```python
from build123d import *

# Parameters (mm, degrees)
SKETCH1_R                  = 20.6375
SKETCH1_R_2                = 17.4625
BOSS_EXTRUDE1_DEPTH        = 152.4
BOSS_EXTRUDE2_START        = -6.35
SKETCH2_R                  = 30.1625
SKETCH2_R_2                = 17.4625
BOSS_EXTRUDE2_DEPTH        = 6.35
F_10_32_TAPPED_HOLE1_D     = 4.0386
F_10_32_TAPPED_HOLE1_DEPTH = 6.35


with BuildPart() as part:
    # Sketch1 → Boss-Extrude1 (new body)
    with BuildSketch(Plane(origin=(0, 0, 0), x_dir=(1, 0, 0), z_dir=(0, 1, 0))):
        with Locations(Location((0, 0, 0), (0, 0, 90))):
            Circle(SKETCH1_R)
        with Locations(Location((0, 0, 0), (0, 0, 90))):
            Circle(SKETCH1_R_2, mode=Mode.SUBTRACT)
    extrude(amount=BOSS_EXTRUDE1_DEPTH)

    # Sketch2 → Boss-Extrude2 (add)
    with BuildSketch(Plane(origin=(0, 152.4, 0), x_dir=(1, 0, 0), z_dir=(0, 1, 0)).offset(BOSS_EXTRUDE2_START)):
        with Locations(Location((0, 0, 0), (0, 0, 270))):
            Circle(SKETCH2_R)
        with Locations(Location((0, 0, 0), (0, 0, 90))):
            Circle(SKETCH2_R_2, mode=Mode.SUBTRACT)
    extrude(amount=BOSS_EXTRUDE2_DEPTH)

    # #10-32 Tapped Hole1
    with Locations(Plane(origin=(0, 152.4, 0), x_dir=(1, 0, 0), z_dir=(0, 1, 0))):
        with Locations((-23.8125, 0), (0, 23.8125), (23.8125, 0), (0, -23.8125), (0, 0)):
            Hole(F_10_32_TAPPED_HOLE1_D / 2, depth=F_10_32_TAPPED_HOLE1_DEPTH)


solid = part.part
```
Here's how the part is built. I have some questions about the finished solid (model axes, mm). A direction names the side the tool comes from. Coordinates: 2 decimals unless noted, no trailing zeros. Write each loop counter-clockwise with the first axis right and the second up, starting at its lowest first coordinate (ties: lowest second). Pieces come first, ordered by that corner, then holes. Notation, with made-up numbers: (18, -26) -> (51, -26) arc R12 cw to (51, -10) -> close; hole circle Ø7 at (70, -31). An arc over 180 degrees is marked (long way). Use a Markdown table: item, result. Add a question column.
(1) If we section it at A-A, the plane z = 0: Write out the boundary of the cut face in (x, y), and give its area (3 significant figures).
(2) If we section it at B-B, the plane x = 11: Write out the boundary of the cut face in (y, z).
(3) Please list where these lines run through material, in increasing order: line 1 (Z direction, x = 0.5, y = 35); line 2 (Y direction, x = 24.5, z = -13); line 3 (Z direction, x = 5.5, y = 23).
(4) For faces 1 (the cylindrical face through (17, 75, 4)), 2 (the cylindrical face through (-20.46, 72, 2.69)), which set-ups out of +Z, -Z, +X, -X, +Y, -Y let a thin tool reach every point of the face, with its end or its side?
(5) If we section it at D-D, the plane x = -8: Write out the boundary of the cut face in (y, z), and give its area (3 significant figures).
(6) If we section it at C-C, the plane y = 82: Write out the boundary of the cut face in (x, z) (1 decimal), and give its area (3 significant figures).
(7) I'm going to push flat-ended pins straight in: P1, Ø10, axis at x = -20, y = 29, coming from the -Z side; P2, Ø5.5, axis at x = 0, z = 23.81, coming from the -Y side; P3, Ø3, axis at x = 10, y = 52, coming from the -Z side; P4, Ø5.5, axis at x = -23.81, z = 0, coming from the +Y side. Where does each tip first touch, or does it pass through?
(8) We'd pull the mould along X, two halves only. Please class faces 3 (the flat face through (-5, 0, 17)), 4 (the cylindrical face through (1.326, 149.181, -30.133)), 5 (the cylindrical face through (0.44, 149.18, -21.84)): +X half, -X half, draft (parallel to the pull), parting line (faces both ways), or undercut.
Outcome:
| question | item | result |
|---|---|---|
| 1 | outline | (-30.16, 146.05) -> (-25.83, 146.05) -> (-25.83, 152.4) -> (-30.16, 152.4) -> close; (-21.79, 146.05) -> (-20.64, 146.05) -> (-20.64, 0) -> (-17.46, 0) -> (-17.46, 152.4) -> (-21.79, 152.4) -> close; (17.46, 0) -> (20.64, 0) -> (20.64, 146.05) -> (21.79, 146.05) -> (21.79, 152.4) -> (17.46, 152.4) -> close; (25.83, 146.05) -> (30.16, 146.05) -> (30.16, 152.4) -> (25.83, 152.4) -> close |
| 1 | area | 1,040 mm^2 |
| 2 | outline | (0, -17.46) -> (146.05, -17.46) -> (146.05, -28.09) -> (152.4, -28.09) -> (152.4, -13.56) -> (0, -13.56) -> close; (0, 13.56) -> (152.4, 13.56) -> (152.4, 28.09) -> (146.05, 28.09) -> (146.05, 17.46) -> (0, 17.46) -> close |
| 3 | line 1 | z = -20.63 to -17.46, 17.46 to 20.63 |
| 3 | line 2 | y = 146.05 to 152.4 |
| 3 | line 3 | z = -19.89 to -16.57, 16.57 to 19.89 |
| 4 | face 1 | +Y, -Y |
| 4 | face 2 | -Y |
| 5 | outline | (0, -19.02) -> (146.05, -19.02) -> (146.05, -29.08) -> (152.4, -29.08) -> (152.4, -15.52) -> (0, -15.52) -> close; (0, 15.52) -> (152.4, 15.52) -> (152.4, 29.08) -> (146.05, 29.08) -> (146.05, 19.02) -> (0, 19.02) -> close |
| 5 | area | 1,200 mm^2 |
| 6 | outline | circle Ø41.3 at (0, 0); hole circle Ø34.9 at (0, 0) |
| 6 | area | 380 mm^2 |
| 7 | P1 | stops at z = -14.17 |
| 7 | P2 | stops at y = 146.05 |
| 7 | P3 | stops at z = -18.81 |
| 7 | P4 | stops at y = 152.4 |
| 8 | face 3 | draft |
| 8 | face 4 | parting line |
| 8 | face 5 | undercut |
